```python
from build123d import *

# Parameters (mm, degrees)
SKETCH_1_W      = 60
SKETCH_1_H      = 10
EXTRUDE_1_DEPTH = 2.5
EXTRUDE_START   = 25
SKETCH_2_W      = 10
SKETCH_2_H      = 20
EXTRUDE_2_DEPTH = 5
SKETCH_5_W      = 10
SKETCH_5_H      = 10
EXTRUDE_3_DEPTH = 10


with BuildPart() as part:
    # 草图1 → 凸台-拉伸1 (new body)
    with BuildSketch(Plane(origin=(0, 0, 0), x_dir=(1, 0, 0), z_dir=(0, 1, 0))):
        Rectangle(SKETCH_1_W, SKETCH_1_H)
    extrude(amount=EXTRUDE_1_DEPTH)

    # 草图2 → 凸台-拉伸2 (add)
    with BuildSketch(Plane(origin=(0, 0, 0), x_dir=(0, 0, -1), z_dir=(1, 0, 0)).offset(EXTRUDE_START)):
        with Locations((0, -7.5)):
            Rectangle(SKETCH_2_W, SKETCH_2_H)
    extrude(amount=EXTRUDE_2_DEPTH)

    # 草图5 → 凸台-拉伸3 (add)
    with BuildSketch(Plane.ZY.offset(-25)):
        with Locations((0, -7.5)):
            Rectangle(SKETCH_5_W, SKETCH_5_H)
    extrude(amount=EXTRUDE_3_DEPTH)


solid = part.part
```
Read the model definition and answer for the solid it produces. Units are mm, in the model's axes. A direction names the side the tool comes from. Give positions to 0.01 mm unless a question says otherwise; leave off trailing zeros. Write each loop counter-clockwise with the first axis right and the second up, starting at its lowest first coordinate (ties: lowest second). Pieces come first, ordered by that corner, then holes. Notation, with made-up numbers: (33.25, 36.5) -> (41.25, 36.5) arc R15 ccw to (41.25, 63.5) -> close; hole circle Ø6 at (86, 41). An arc over 180 degrees is marked (long way). Answer in a Markdown table with one row per item.
1) Straight lines are drawn through the part: line 1 (Y direction, x = 23.5, z = -2.75); line 2 (X direction, y = -12.25, z = 4); line 3 (Y direction, x = -1, z = 4). For each, find the intervals that lie inside material, in ascending order. Write a range as [from, to].
Results list:
| item | result |
|---|---|
| line 1 | [-12.5, -2.5], [0, 2.5] |
| line 2 | [15, 30] |
| line 3 | [0, 2.5] |
2) Section B-B on x = 8.5 is taken. Give the vertices of the cut face in (y, z).
Results list:
| item | result |
|---|---|
| outline | (0, -5) -> (2.5, -5) -> (2.5, 5) -> (0, 5) -> close |
3) Determine the mould class of faces 1 (the flat face through (-30, 1, 0)), 2 (the flat face through (20, -12.5, 0)), 3 (the flat face through (25, -1, 0)) for opening direction Y: released by +Y, released by -Y, zero draft, split by the parting line, or undercut.
Results list:
| item | result |
|---|---|
| face 1 | zero draft |
| face 2 | released by -Y |
| face 3 | undercut |
4) A tool of negligible diameter and unlimited length cuts with its end or side. For faces 4 (the flat face through (25, -15, 0)), 5 (the flat face through (20, -2.5, 0)), 6 (the flat face through (30, -7, 0)), from which of +Z, -Z, +X, -X, +Y, -Y can it reach the whole face along a straight path? Write none if from no direction.
Results list:
| item | result |
|---|---|
| face 4 | +Z, -Z, -X, -Y |
| face 5 | +Z, -Z, -X |
| face 6 | +Z, -Z, +X, +Y, -Y |
5) Each of these flat-tipped pins is pushed along its axis until it touches: pin 1 Ø4 at (x, y) = (0.5, -3) entering from -Z; pin 2 Ø4 at (y, z) = (-14, -1) entering from -X; pin 3 Ø1.2 at (y, z) = (-1.5, 0) entering from -X; pin 4 Ø5 at (x, z) = (19.5, 1.5) entering from -Y. Where does it stop, or does it pass through?
Results list:
| item | result |
|---|---|
| pin 1 | through |
| pin 2 | x = 15 |
| pin 3 | x = 25 |
| pin 4 | y = -12.5 |
6) Section C-C on y = -4.25 is taken. Give the vertices of the cut face in (x, z), plus the area to 3 significant figures.
Results list:
| item | result |
|---|---|
| outline | (15, -5) -> (30, -5) -> (30, 5) -> (15, 5) -> close |
| area | 150 mm^2 |
7) Section A-A on z = 3.5 is taken. Give the vertices of the cut face in (x, y), plus the area to 4 significant figures.
Results list:
| item | result |
|---|---|
| outline | (-30, 0) -> (25, 0) -> (25, -2.5) -> (15, -2.5) -> (15, -12.5) -> (25, -12.5) -> (25, -17.5) -> (30, -17.5) -> (30, 2.5) -> (-30, 2.5) -> close |
| area | 337.5 mm^2 |
